Verification items for this drawing (mm, ordinates from the low corner). Coordinates: 2 decimals unless noted, no trailing zeros. Loops run counter-clockwise (first coordinate to the right, second up) from the corner with the lowest first, then second, coordinate; pieces in that order, holes last. Notation, with made-up numbers: M 1,46 L 41,46 A25 ccw 41,82 Z; hole C 9,57.5 d2. An arc over 180 degrees is marked long. Return JSON: item names as keys, results as strings.
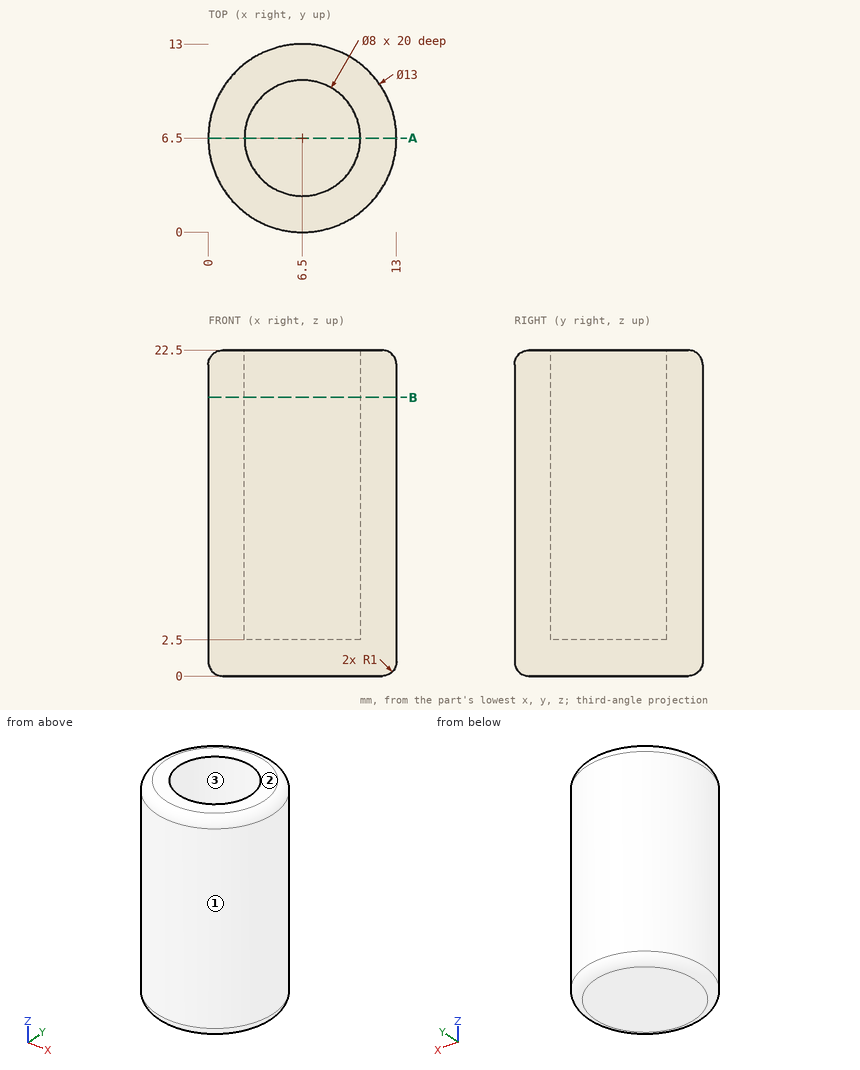
1) Scan lines: line 1 along Y through (x, z) = (6.5, 11.5); line 2 along Z through (x, y) = (7.75, 4); line 3 along X through (y, z) = (6, 9.5). Record each from-to range of solid material in increasing order. Write a range as [from, to].
Answers:
{"line 1": "[0, 2.5], [10.5, 13]", "line 2": "[0, 2.5]", "line 3": "[0.02, 2.53], [10.47, 12.98]"}
2) Draft check along Y on the marked faces 1, 2 and 3. Enter one of: +Y half, -Y half, draft (parallel to the pull), parting line (faces both ways), or undercut.
Answers:
{"face 1": "parting line", "face 2": "draft", "face 3": "undercut"}
3) Go/stop test with flat-tipped pins: pin 1 Ø1 at (x, z) = (6, 2.5) entering from +Y; pin 2 Ø3 at (y, z) = (3.5, 5.5) entering from +X; pin 3 Ø3 at (y, z) = (11.5, 10.5) entering from +X; pin 4 Ø1 at (x, y) = (7, 7.5) entering from +Z. Record where each tip stops, or that it passes through.
Answers:
{"pin 1": "y = 13", "pin 2": "x = 12.82", "pin 3": "x = 11.98", "pin 4": "z = 2.5"}
4) Section check A-A on y = 6.5. Record the cut outline in (x, z).
Answers:
{"outline": "M 0,1 A1 ccw 1,0 L 12,0 A1 ccw 13,1 L 13,21.5 A1 ccw 12,22.5 L 10.5,22.5 L 10.5,2.5 L 2.5,2.5 L 2.5,22.5 L 1,22.5 A1 ccw 0,21.5 Z"}
5) Section check B-B on z = 19.25. Record the cut outline in (x, y), then the cut area to 3 significant figures.
Answers:
{"outline": "C 6.5,6.5 d13; hole C 6.5,6.5 d8", "area": "82.5 mm²"}
